Autodesk Inventor part; units mm, degrees
ref_plane "YZ Plane" through (0, 0, 0) normal (1, 0, 0) x (0, 1, 0)
ref_plane "XZ Plane" through (0, 0, 0) normal (0, 1, 0) x (-1, 0, 0)
ref_plane "XY Plane" through (0, 0, 0) normal (0, 0, 1) x (1, 0, 0)
sketch "Sketch1" plane through (0, 0, 0) normal (0, 1, 0) x (-1, 0, 0)
  line L0 (0, 96.3881) -> (0, -80.6119)
  line L1 (0, -80.6119) -> (7.6619, -80.6119)
  line L2 (7.6619, -80.6119) -> (7.6619, -63.0119)
  line L3 (7.6619, -63.0119) -> (55.6286, -47.1119)
  line L4 (55.6286, -47.1119) -> (55.6286, 62.8881)
  line L5 (55.6286, 62.8881) -> (7.6619, 78.7881)
  line L6 (7.6619, 78.7881) -> (7.6619, 96.3881)
  line L7 (7.6619, 96.3881) -> (0, 96.3881)
  point P0 (0, 0)
  dimension "d0" = 177
  dimension "d1" = 17.6
  dimension "d2" = 17.6
  dimension "d3" = 110
  dimension "d4" = 15.9
extrude "Extrusion1" add sketch "Sketch1" along normal blind 150
sketch "Sketch2" plane through (0, 150, 0) normal (0, 1, 0) x (1, 0, 0)
  line L0 (-7.6619, -78.7881) -> (-7.6619, -96.3881)
  line L1 (-7.6619, -78.7881) -> (0, -78.7881)
  line L2 (0, -96.3881) -> (0, 80.6119)
  line L3 (0, -78.7881) -> (0, -67.7881)
  line L4 (0, -67.7881) -> (-7.6619, -67.7881)
  line L5 (-7.6619, 80.6119) -> (-7.6619, 63.0119)
  line L6 (-7.6619, 63.0119) -> (0, 63.0119)
  line L7 (0, 63.0119) -> (0, 52.0119)
  line L8 (0, 52.0119) -> (-7.6619, 52.0119)
  line L9 (0, -67.7881) -> (0, 52.0119)
  line L10 (-7.6619, -67.7881) -> (-47.625, -54.5411)
  line L11 (-7.6619, 52.0119) -> (-47.625, 38.7649)
  line L12 (-55.6286, -62.8881) -> (-7.6619, -78.7881)
  line L13 (-7.6619, 63.0119) -> (-55.6286, 47.1119)
  line L14 (-47.625, -54.5411) -> (-47.625, 38.7649)
  point P0 (0, 0)
  dimension "d8" = 11
  dimension "d9" = 11
  dimension "d10" = 0
  dimension "d11" = 0
  dimension "d12" = 93.306
extrude "Extrusion2" cut sketch "Sketch2" against normal blind 150
sketch "Sketch3" plane through (0, 0, -80.6119) normal (0, 0, -1) x (-1, 0, 0)
  line L0 (0, 0) -> (0, 150)
  line L1 (0, 135) -> (7.7027, 135)
  line L2 (7.7027, 135) -> (47.625, 122.3)
  line L3 (47.625, 150) -> (47.625, 0)
  line L4 (47.625, 122.3) -> (47.625, 101.6779)
  line L5 (47.625, 101.6779) -> (7.6619, 88.9625)
  line L6 (7.6619, 150) -> (7.6619, 0)
  line L7 (7.6619, 88.9625) -> (0, 88.9625)
  line L8 (0, 135) -> (0, 88.9625)
  line L9 (0, 73.9625) -> (7.7027, 73.9625)
  line L10 (7.7027, 73.9625) -> (47.625, 61.2625)
  line L11 (47.625, 61.2625) -> (47.625, 27.7154)
  line L12 (47.625, 27.7154) -> (7.6619, 15)
  line L13 (7.6619, 15) -> (0, 15)
  line L14 (0, 73.9625) -> (0, 15)
  line L15 (0, 150) -> (7.6619, 150)
  line L16 (0, 0) -> (7.6619, 0)
  point P0 (7.6619, 15)
  point P1 (7.6619, 73.9625)
  point P2 (7.6619, 135)
  dimension "d15" = 72.35
  dimension "d16" = 72.353
  dimension "d18" = 15
  dimension "d19" = 15
  dimension "d20" = 46.0375
  dimension "d22" = 72.353
  dimension "d23" = 72.35
  dimension "d24" = 15
extrude "Extrusion3" cut sketch "Sketch3" against normal blind 1500 contours L6 L9 L10 L3 L12 | L6 L1 L2 L3 L5
fillet "Fillet1" radius 2 8 edges at (-47.625, 122.3, -44.2649) (-47.625, 101.6779, -44.2649) (-47.625, 61.2625, -44.2649) (-47.625, 27.7154, -44.2649) (-47.625, 61.2625, 60.0411) (-47.625, 122.3, 60.0411) (-47.625, 101.6779, 60.0411) (-47.625, 27.7154, 60.0411)
fillet "Fillet2" radius 2 12 edges at (-47.625, 121.5687, 54.5411) (-47.625, 136.15, 54.5411) (-47.625, 60.5312, 54.5411) (-47.625, 102.4092, 54.5411) (-47.625, 28.4467, 54.5411) (-47.625, 13.8577, 54.5411) (-47.625, 136.15, -38.7649) (-47.625, 121.5687, -38.7649) (-47.625, 60.5312, -38.7649) (-47.625, 102.4092, -38.7649) (-47.625, 13.8577, -38.7649) (-47.625, 28.4467, -38.7649)
fillet "Fillet3" radius 2 4 edges at (-7.6619, 75, 96.3881) (-7.6619, 75, -80.6119) (-55.6286, 75, -47.1119) (-55.6286, 75, 62.8881)
sketch "Sketch4" plane through (-7.6619, 15, -52.0119) normal (-1, 0, 0) x (0, 0, 1)
  line L0 (130.8, 135) -> (146.4, 135)
  line L1 (139.9, 135) -> (139.9, -14.5366)
  line L2 (-20.1, 135) -> (-20.1, -15)
  line L3 (-26.6, -15) -> (-26.6, 135)
  line L4 (-26.6, -15) -> (-11, -15)
  line L5 (148.4, -15) -> (148.4, 135)
  circle A0 centre (-20.1, 127.5) radius 2.475
  line L6 (-26.6, 135) -> (-11, 135)
  circle A1 centre (-20.1, 66.4625) radius 2.475
  circle A2 centre (-20.1, -7.5) radius 2.475
  line L7 (-10.9865, 58.9625) -> (0.0135, 58.9625)
  point P0 (52.0119, -15)
  dimension "d30" = 160
  dimension "d31" = 150
  dimension "d32" = 0
  dimension "d33" = 8.5
  dimension "d34" = 4.95
  dimension "d35" = 7.5
  dimension "d36" = 7.5
  dimension "d37" = 7.5
extrude "Extrusion4" cut sketch "Sketch4" against normal blind 1500 contours A0 L2 | L2 A0 | A1 L2 | L2 A1 | A2 L2 | L2 A2
ref_plane "Work Plane1" through (-221.551, 135, 7.8881) normal (0, 0, -1) x (0, -1, 0)
mirror "Mirror1" about plane through (-221.551, 135, 7.8881) normal (0, 0, -1) of "Extrusion4"
properties part number "SpotAttachment"
Read the model definition and answer for the solid it produces. Units are mm, in the model's axes. A direction names the side the tool comes from. Give positions to 0.01 mm unless a question says otherwise; leave off trailing zeros. Write each loop counter-clockwise with the first axis right and the second up, starting at its lowest first coordinate (ties: lowest second). Pieces come first, ordered by that corner, then holes. Notation, with made-up numbers: (-1, 14) -> (19, 14) arc R20 cw to (19, 25) -> close; hole circle Ø3 at (31, 75.25). An arc over 180 degrees is marked (long way). Answer in a Markdown table with one row per item.
1) Section B-B on x = -43 is taken. Give the vertices of the cut face in (y, z).
Results list:
| item | result |
|---|---|
| outline | (0, -51.3) -> (26.24, -51.3) -> (26.24, -40.3) -> (0, -40.3) -> close; (0, 56.07) -> (26.24, 56.07) -> (26.24, 67.07) -> (0, 67.07) -> close; (62.73, -51.3) -> (100.21, -51.3) -> (100.21, -40.3) -> (62.73, -40.3) -> close; (62.73, 56.07) -> (100.21, 56.07) -> (100.21, 67.07) -> (62.73, 67.07) -> close; (123.77, -51.3) -> (150, -51.3) -> (150, -40.3) -> (123.77, -40.3) -> close; (123.77, 56.07) -> (150, 56.07) -> (150, 67.07) -> (123.77, 67.07) -> close |
2) Determine the mould class of faces 4 (the flat face through (-36.46, 73.95, 69.24)), 5 (the flat face through (0, 74, 82)), 6 (the cylindrical face through (-3.885, 140.084, -72.648)) for opening direction Z: released by +Z, released by -Z, zero draft, split by the parting line, or undercut.
Results list:
| item | result |
|---|---|
| face 4 | released by +Z |
| face 5 | zero draft |
| face 6 | undercut |
3) Section D-D on x = -23.5 is taken. Give the vertices of the cut face in (y, z), plus the area to 3 significant figures.
Results list:
| item | result |
|---|---|
| outline | (0, -57.76) -> (20.04, -57.76) -> (20.04, -46.76) -> (0, -46.76) -> close; (0, 62.54) -> (20.04, 62.54) -> (20.04, 73.54) -> (0, 73.54) -> close; (68.94, -57.76) -> (94, -57.76) -> (94, -46.76) -> (68.94, -46.76) -> close; (68.94, 62.54) -> (94, 62.54) -> (94, 73.54) -> (68.94, 73.54) -> close; (129.97, -57.76) -> (150, -57.76) -> (150, -46.76) -> (129.97, -46.76) -> close; (129.97, 62.54) -> (150, 62.54) -> (150, 73.54) -> (129.97, 73.54) -> close |
| area | 1,430 mm^2 |
4) Section C-C on z = 9 is taken. Give the vertices of the cut face in (x, y) (3 decimals), plus the area to 3 significant figures.
Results list:
| item | result |
|---|---|
| outline | (-55.629, 0) -> (-47.625, 0) -> (-47.625, 150) -> (-55.629, 150) -> close |
| area | 1,200 mm^2 |
5) Each of these flat-tipped pins is pushed along its axis until it touches: pin 1 Ø5.5 at (y, z) = (142.5, 87.89) entering from -X; pin 2 Ø4 at (y, z) = (81.46, -72.11) entering from -X; pin 3 Ø1 at (y, z) = (72.5, 39.5) entering from +X (3 decimals); pin 4 Ø1 at (x, y) = (-6.5, 38) entering from +Z. Where does it stop, or does it pass through?
Results list:
| item | result |
|---|---|
| pin 1 | x = -7.66 |
| pin 2 | through |
| pin 3 | x = -47.625 |
| pin 4 | z = 96.36 |
6) Straight lines are drawn through the part: line 1 (Z direction, x = -4.25, y = 7.5); line 2 (X direction, y = 40.5, z = -58.5); line 3 (Z direction, x = -30.5, y = 128.5). For each, find the intervals that lie inside material, in ascending order. Write a range as [from, to].
Results list:
| item | result |
|---|---|
| line 1 | [-80.61, -74.59], [-69.64, -52.01], [67.79, 85.41], [90.36, 96.39] |
| line 2 | [-7.66, 0] |
| line 3 | [-55.44, -44.44], [60.22, 71.22] |
7) Section A-A on y = 142.5 is taken. Give the vertices of the cut face in (x, z) (3 decimals), plus the area to 3 significant figures.
Results list:
| item | result |
|---|---|
| outline | (-55.629, -45.668) arc R2 ccw to (-54.258, -47.566) -> (-7.662, -63.012) -> (-7.662, -69.637) -> (0, -69.637) -> (0, -52.012) -> (-7.662, -52.012) -> (-46.254, -39.219) arc R2 cw to (-47.625, -37.321) -> (-47.625, 53.097) arc R2 cw to (-46.254, 54.995) -> (-7.662, 67.788) -> (0, 67.788) -> (0, 85.413) -> (-7.662, 85.413) -> (-7.662, 78.788) -> (-54.258, 63.342) arc R2 ccw to (-55.629, 61.444) -> close; (-7.662, -78.612) arc R2 ccw to (-5.662, -80.612) -> (0, -80.612) -> (0, -74.587) -> (-7.662, -74.587) -> close; (-7.662, 90.363) -> (0, 90.363) -> (0, 96.388) -> (-5.662, 96.388) arc R2 ccw to (-7.662, 94.388) -> close |
| area | 2,140 mm^2 |
8) A tool of negligible diameter and unlimited length cuts with its end or side. For faces 1 (the flat face through (-26.7, 10.8, -45.7)), 2 (the cylindrical face through (-3.88, 144.7, 86.75)), 3 (the flat face through (-27.217, 21.222, -51.286)), from which of +Z, -Z, +X, -X, +Y, -Y can it reach the whole face along a straight path? Write none if from no direction.
Results list:
| item | result |
|---|---|
| face 1 | +X, +Y, -Y |
| face 2 | +X, -X |
| face 3 | +Z, -Z |
